from build123d import *

# Parameters (mm, degrees)
F0_R     = 7.9375
F1_DEPTH = 101.6
F3_D     = 5.1054
F3_DEPTH = 16.51
F3_TIP   = 1.5338169022
F5_D     = 5.1054
F5_DEPTH = 16.51
F5_TIP   = 1.5338169022


with BuildPart() as f1:
    # F0 (on Top) → F1 (new body, symmetric)
    with BuildSketch(Plane.XY):
        Circle(F0_R)
    extrude(amount=F1_DEPTH, both=True)

    # F3
    with Locations(Plane.XY.offset(101.6)):
        with Locations((0, 0)):
            Hole(F3_D / 2, depth=F3_DEPTH)
            with Locations((0, 0, -(F3_DEPTH + F3_TIP / 2))):  # 118° drill point
                Cone(0, F3_D / 2, F3_TIP, mode=Mode.SUBTRACT)

    # F5
    with Locations(Plane(origin=(0, 0, -101.6), x_dir=(1, 0, 0), z_dir=(0, 0, -1))):
        with Locations((0, 0)):
            Hole(F5_D / 2, depth=F5_DEPTH)
            with Locations((0, 0, -(F5_DEPTH + F5_TIP / 2))):  # 118° drill point
                Cone(0, F5_D / 2, F5_TIP, mode=Mode.SUBTRACT)


solid = f1.part
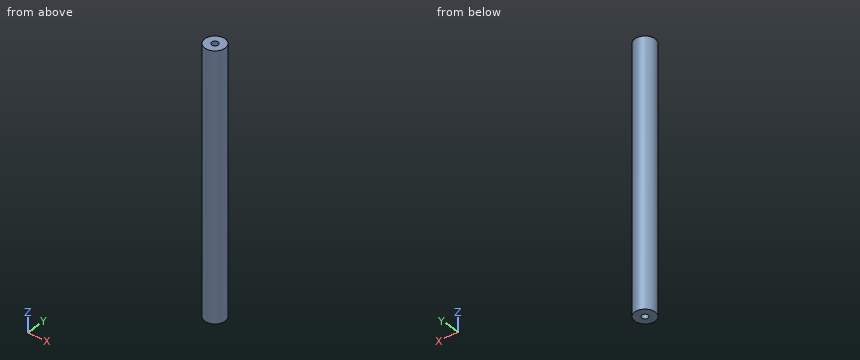
Verification items for the finished model (mm, model axes). Round coordinates to 2 decimals unless told otherwise and drop trailing zeros. Loops run counter-clockwise (first coordinate to the right, second up) from the corner with the lowest first, then second, coordinate; pieces in that order, holes last. Notation, with made-up numbers: (-7, 55.25) - (21, 55.25) arc R16 cw to (21, 63.25) - close; hole circle Ø5 at (16.25, 55). An arc over 180 degrees is marked (long way). Write item = value, one per line.
Q1. Sectioned sample at C-C on y = 4.75. Record the boundary of the cut face in (x, z).
Here are the results:
outline = (-6.36, -101.6) - (6.36, -101.6) - (6.36, 101.6) - (-6.36, 101.6) - close
Q2. Depth check by flat-ended pin: pin 1 (3 mm diameter, centred on x = 5, z = 73.5, fed in from +Y); pin 2 (2 mm diameter, centred on y = -4.5, z = 4.5, fed in from -X); pin 3 (1 mm diameter, centred on x = 6.5, z = -79.5, fed in from -Y); pin 4 (3 mm diameter, centred on x = -1, z = -16.5, fed in from +Y). Enter the tip coordinate at first touch or a pass-through.
Here are the results:
pin_1 = 7.12
pin_2 = -7.12
pin_3 = -5.2
pin_4 = 7.94
Q3. Material ranges on L1, parallel to Y at x = 0, z = 97.75; L2, parallel to Y at x = -0.5, z = 35; L3, parallel to Y at x = -5.25, z = 48.5, recorded low to high.
Here are the results:
L1 = -7.94 to -2.55, 2.55 to 7.94
L2 = -7.92 to 7.92
L3 = -5.95 to 5.95
Q4. Sectioned sample at A-A on z = -59. Record the boundary of the cut face in (x, y) (1 decimal), plus the area to 3 significant figures.
Here are the results:
outline = circle Ø15.9 at (0, 0)
area = 198 mm^2
Q5. Sectioned sample at B-B on x = 6. Record the boundary of the cut face in (y, z).
Here are the results:
outline = (-5.2, -101.6) - (5.2, -101.6) - (5.2, 101.6) - (-5.2, 101.6) - close
